Design review of the part shown in the three views and the two pictorial views. Dimensions are in mm from the part's minimum x, y and z. Round coordinates to 2 decimals unless told otherwise and drop trailing zeros. Order: outer loops, then holes, each group sorted by start corner. A loop starts at its lowest first (then second) coordinate and runs counter-clockwise, first axis right, second up. Notation, with made-up numbers: M 33,73 L 78,73 A13 cw 78,87 Z; hole C 49.5,49.25 d5. An arc over 180 degrees is marked long. Write each question's results on one line, items separated by ' | '. Start each with the question number.
Item 1: Clearance check with a flat-ended pin moving along its axis: pin 1 (1.9 mm diameter, centred on x = 2.59, z = 2.19, fed in from -Y). State where the tip first meets the part, or that it passes through.
Item 2: Wall thickness on line 1 (Z direction, x = 2.59, y = 0.85); line 2 (X direction, y = 0.6, z = 28.1): over which ranges is each line inside the solid? List them lowest first. Write a range as [from, to].
Item 3: Take a section at A-A, the plane x = 2.59. Write out the cut boundary in (y, z).
Item 4: Take a section at B-B, the plane z = 2.19. Write out the cut boundary in (x, y), plus the area to 3 significant figures.
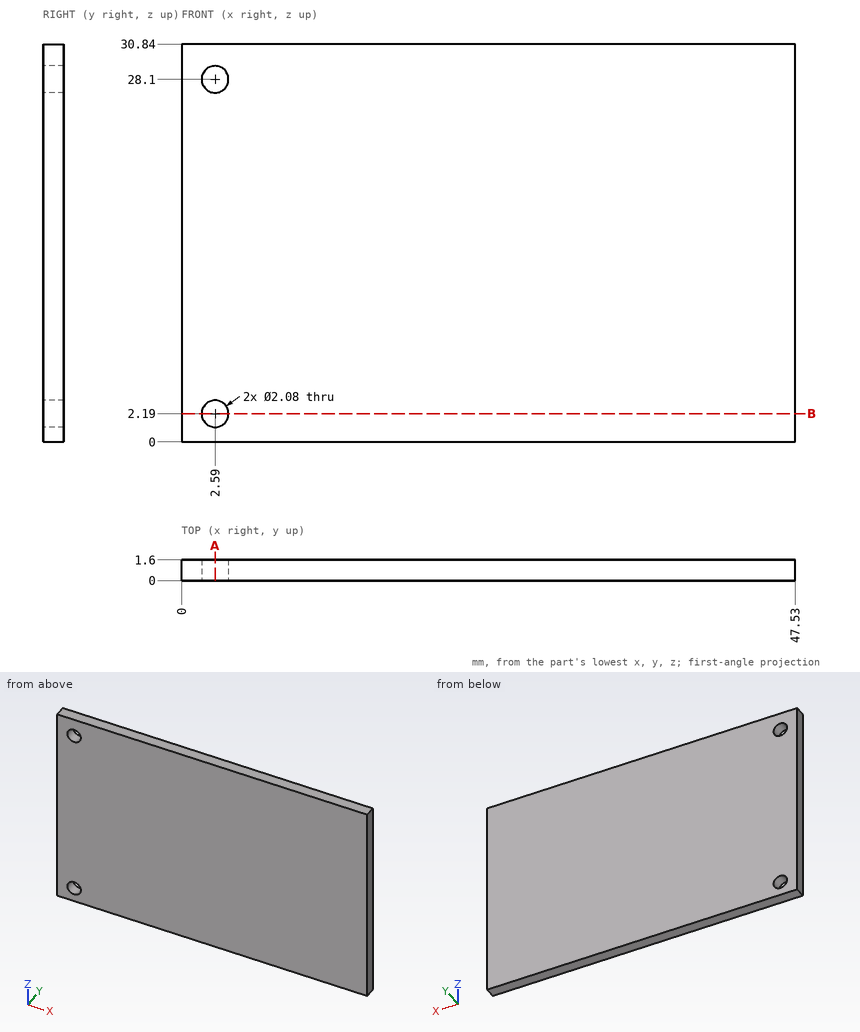
Results list:
1) pin 1: through
2) line 1: [0, 1.15], [3.23, 27.06], [29.14, 30.84] | line 2: [0, 1.55], [3.63, 47.53]
3) outline: M 0,0 L 1.6,0 L 1.6,1.15 L 0,1.15 Z; M 0,3.23 L 1.6,3.23 L 1.6,27.06 L 0,27.06 Z; M 0,29.14 L 1.6,29.14 L 1.6,30.84 L 0,30.84 Z
4) outline: M 0,0 L 1.55,0 L 1.55,1.6 L 0,1.6 Z; M 3.63,0 L 47.53,0 L 47.53,1.6 L 3.63,1.6 Z | area: 72.7 mm²
